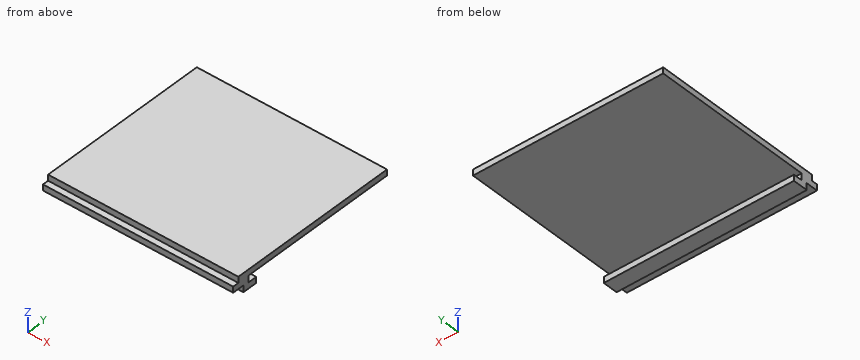
```python
from build123d import *

# Parameters (mm, degrees)
BOSS_EXTRUDE1_DEPTH = 406.4
SKETCH3_W           = 12.7
SKETCH3_H           = 12.7
BOSS_EXTRUDE2_DEPTH = 406.4
SKETCH4_W           = 12.7
SKETCH4_H           = 25.4
BOSS_EXTRUDE3_DEPTH = 406.4


with BuildPart() as part:
    # Sketch2 → Boss-Extrude1 (new body)
    with BuildSketch(Plane(origin=(0, 0, 0), x_dir=(0, 0, -1), z_dir=(1, 0, 0))):
        Polygon((0, 0), (39.639393939, 0), (39.639393939, 31.75), (26.939393939, 31.75), (26.939393939, 12.7), (12.7, 12.7), (12.7, 355.6), (0, 355.6), align=None)
    extrude(amount=BOSS_EXTRUDE1_DEPTH)

    # Sketch3 → Boss-Extrude2 (add)
    with BuildSketch(Plane(origin=(406.4, 0, 0), x_dir=(0, 0, -1), z_dir=(1, 0, 0))):
        with Locations((6.35, -6.35)):
            Rectangle(SKETCH3_W, SKETCH3_H)
    extrude(amount=-BOSS_EXTRUDE2_DEPTH)

    # Sketch4 → Boss-Extrude3 (add)
    with BuildSketch(Plane(origin=(406.4, 0, 0), x_dir=(0, 0, -1), z_dir=(1, 0, 0))):
        with Locations((19.05, -12.7)):
            Rectangle(SKETCH4_W, SKETCH4_H)
    extrude(amount=-BOSS_EXTRUDE3_DEPTH)


solid = part.part
```
Here's how the part is built. I have some questions about the finished solid (model axes, mm). Give positions to 0.01 mm unless a question says otherwise; leave off trailing zeros. Loops run counter-clockwise (first coordinate to the right, second up) from the corner with the lowest first, then second, coordinate; pieces in that order, holes last. Notation, with made-up numbers: (2, 68.5) -> (23, 68.5) arc R17 ccw to (23, 101.5) -> close; hole circle Ø10 at (21.5, 12). An arc over 180 degrees is marked (long way). Use one line per item in the form item = value. Start each with the question number.
1) Please list where these lines run through material, in increasing order: line 1 along Y through (x, z) = (268, -30); line 2 along Z through (x, y) = (92, 281); line 3 along Y through (x, z) = (340.5, -7.5).
2) Imagine slicing it at A-A (x = 58.5). Please give me the cut outline in (y, z), then the cut area to 3 significant figures.
3) For P1, Ø12, axis at x = 364.5, y = 42, coming from the -Z side; P2, Ø6.5, axis at x = 108, z = -8.5, coming from the -Y side; P3, Ø3, axis at x = 82, z = -29, coming from the -Y side, each with a flat end and sliding along its axis, tell me the tip position at first contact or that it passes through.
4) Imagine slicing it at B-B (z = -19). Please give me the cut outline in (x, y), then the cut area to 3 significant figures.
5) Imagine slicing it at C-C (y = 58). Please give me the cut outline in (x, z), then the cut area to 3 significant figures.
Check values:
q1.line_1 = 0 to 31.75
q1.line_2 = -12.7 to 0
q1.line_3 = -12.7 to 355.6
q2.outline = (-25.4, -25.4) -> (0, -25.4) -> (0, -39.64) -> (31.75, -39.64) -> (31.75, -26.94) -> (12.7, -26.94) -> (12.7, -12.7) -> (355.6, -12.7) -> (355.6, 0) -> (-12.7, 0) -> (-12.7, -12.7) -> (-25.4, -12.7) -> close
q2.area = 5,580 mm^2
q3.P1 = -12.7
q3.P2 = -12.7
q3.P3 = 0
q4.outline = (0, -25.4) -> (406.4, -25.4) -> (406.4, 12.7) -> (0, 12.7) -> close
q4.area = 15,500 mm^2
q5.outline = (0, -12.7) -> (406.4, -12.7) -> (406.4, 0) -> (0, 0) -> close
q5.area = 5,160 mm^2
